Input: part model. Units: mm. Frame: model coordinates. A direction names the side the tool comes from. Coordinates: 2 decimals unless noted, no trailing zeros. Loops run counter-clockwise (first coordinate to the right, second up) from the corner with the lowest first, then second, coordinate; pieces in that order, holes last.
```python
from build123d import *

# Parameters (mm, degrees)
SKETCH1_W           = 178
SKETCH1_H           = 178
SKETCH1_R           = 3.57
BOSS_EXTRUDE1_DEPTH = 0.8
FILLET1_R           = 13
CUT_EXTRUDE1_DEPTH  = 10


with BuildPart() as part:
    # Sketch1 → Boss-Extrude1 (new body)
    with BuildSketch(Plane.XY):
        with Locations((89, -89)):
            Rectangle(SKETCH1_W, SKETCH1_H)
        with Locations((25.5, -25.5)):
            Circle(SKETCH1_R, mode=Mode.SUBTRACT)
        with Locations((152.5, -25.5)):
            Circle(SKETCH1_R, mode=Mode.SUBTRACT)
        with Locations((152.5, -152.5)):
            Circle(SKETCH1_R, mode=Mode.SUBTRACT)
        with Locations((25.5, -152.5)):
            Circle(SKETCH1_R, mode=Mode.SUBTRACT)
    extrude(amount=BOSS_EXTRUDE1_DEPTH)

    # Fillet1
    fillet1_edges = [part.edges().sort_by_distance(p)[0] for p in [
        (0, 0, 0.4),
        (178, 0, 0.4),
        (178, -178, 0.4),
        (0, -178, 0.4),
    ]]
    fillet(fillet1_edges, radius=FILLET1_R)

    # Sketch2 → Cut-Extrude1 (cut)
    with BuildSketch(Plane.XY.offset(0.8)):
        with BuildLine():
            Line((88.25, -61.510229175), (88.25, -60.009699898))
            ThreePointArc((88.25, -60.009699898), (77.902180461, -62.207493557), (69.031092295, -67.970432123))
            Line((69.031092295, -67.970432123), (70.092126722, -69.031466551))
            ThreePointArc((70.092126722, -69.031466551), (78.47620561, -63.593312856), (88.25, -61.510229175))
        make_face()
        with BuildLine():
            ThreePointArc((108.968907705, -67.970432123), (100.097819539, -62.207493557), (89.75, -60.009699898))
            Line((89.75, -60.009699898), (89.75, -61.510229175))
            ThreePointArc((89.75, -61.510229175), (99.52379439, -63.593312856), (107.907873278, -69.031466551))
            Line((107.907873278, -69.031466551), (108.968907705, -67.970432123))
        make_face()
        with BuildLine():
            ThreePointArc((117.990300102, -88.25), (115.792506443, -77.902180461), (110.029567877, -69.031092295))
            Line((110.029567877, -69.031092295), (108.968533449, -70.092126722))
            ThreePointArc((108.968533449, -70.092126722), (114.406687144, -78.47620561), (116.489770825, -88.25))
            Line((116.489770825, -88.25), (117.990300102, -88.25))
        make_face()
        with BuildLine():
            ThreePointArc((89.75, -117.990300102), (100.097819539, -115.792506443), (108.968907705, -110.029567877))
            Line((108.968907705, -110.029567877), (107.907873278, -108.968533449))
            ThreePointArc((107.907873278, -108.968533449), (99.52379439, -114.406687144), (89.75, -116.489770825))
            Line((89.75, -116.489770825), (89.75, -117.990300102))
        make_face()
        with BuildLine():
            ThreePointArc((110.029567877, -108.968907705), (115.792506443, -100.097819539), (117.990300102, -89.75))
            Line((117.990300102, -89.75), (116.489770825, -89.75))
            ThreePointArc((116.489770825, -89.75), (114.406687144, -99.52379439), (108.968533449, -107.907873278))
            Line((108.968533449, -107.907873278), (110.029567877, -108.968907705))
        make_face()
        with BuildLine():
            Line((69.031466551, -70.092126722), (67.970432123, -69.031092295))
            ThreePointArc((67.970432123, -69.031092295), (62.207493557, -77.902180461), (60.009699898, -88.25))
            Line((60.009699898, -88.25), (61.510229175, -88.25))
            ThreePointArc((61.510229175, -88.25), (63.593312856, -78.47620561), (69.031466551, -70.092126722))
        make_face()
        with BuildLine():
            Line((61.510229175, -89.75), (60.009699898, -89.75))
            ThreePointArc((60.009699898, -89.75), (62.207493557, -100.097819539), (67.970432123, -108.968907705))
            Line((67.970432123, -108.968907705), (69.031466551, -107.907873278))
            ThreePointArc((69.031466551, -107.907873278), (63.593312856, -99.52379439), (61.510229175, -89.75))
        make_face()
        with BuildLine():
            Line((70.092126722, -108.968533449), (69.031092295, -110.029567877))
            ThreePointArc((69.031092295, -110.029567877), (77.902180461, -115.792506443), (88.25, -117.990300102))
            Line((88.25, -117.990300102), (88.25, -116.489770825))
            ThreePointArc((88.25, -116.489770825), (78.47620561, -114.406687144), (70.092126722, -108.968533449))
        make_face()
    extrude(amount=-CUT_EXTRUDE1_DEPTH, mode=Mode.SUBTRACT)


solid = part.part
```
Item 1: Mould query, pull axis X, two halves, no side actions, for faces 1 (the face through (3.707, -3.909, 0.406)), 2 (the face through (174.091, -174.293, 0.406)), 3 (the face through (77.765, -115.735, 0.406)). Classes: +X half, -X half, draft (parallel to the pull), parting line (faces both ways), or undercut.
Result:
face 1: -X half
face 2: +X half
face 3: undercut
Item 2: Reachability of faces 4 (the face through (100.235, -62.265, 0.406)), 5 (the face through (174.091, -3.707, 0.406)) from +Z, -Z, +X, -X, +Y, -Y: full face, straight path, thin tool, end or side. Return the list, or none.
Result:
face 4: +Z, -Z
face 5: +Z, -Z, +X, +Y
Item 3: Section query B-B (y = -152.5). Output: boundary loops of the cut face in (x, z), then the cut area to 3 significant figures.
Result:
outline: (0, 0) - (21.93, 0) - (21.93, 0.8) - (0, 0.8) - close; (29.07, 0) - (148.93, 0) - (148.93, 0.8) - (29.07, 0.8) - close; (156.07, 0) - (178, 0) - (178, 0.8) - (156.07, 0.8) - close
area: 131 mm2
Item 4: Section query C-C (z = 0.5). Count the separate pieces of the cut face and the enclosed holes in it, then the cut area to 3 significant figures.
Result:
separate pieces: 1
enclosed holes: 12
area: 31,100 mm2
Item 5: Section query A-A (x = 152.5). Output: boundary loops of the cut face in (y, z), then the cut area to 3 significant figures.
Result:
outline: (-178, 0) - (-156.07, 0) - (-156.07, 0.8) - (-178, 0.8) - close; (-148.93, 0) - (-29.07, 0) - (-29.07, 0.8) - (-148.93, 0.8) - close; (-21.93, 0) - (0, 0) - (0, 0.8) - (-21.93, 0.8) - close
area: 131 mm2
Item 6: Line query: L1, parallel to X at y = -152.5, z = 0.6; L2, parallel to Y at x = 152.5, z = 0.5; L3, parallel to Y at x = 87, z = 0.75. Output: solid intervals per line, ascending.
Result:
L1: x = 0 to 21.93, 29.07 to 148.93, 156.07 to 178
L2: y = -178 to -156.07, -148.93 to -29.07, -21.93 to 0
L3: y = -178 to -117.93, -116.43 to -61.57, -60.07 to 0
